Check sheet for the modelled part. Datum: model origin and axes. Units: mm. A direction names the side the tool comes from. Round coordinates to 2 decimals unless told otherwise and drop trailing zeros. Write each loop counter-clockwise with the first axis right and the second up, starting at its lowest first coordinate (ties: lowest second). Pieces come first, ordered by that corner, then holes.
Item 1: Set-up check for faces 4 (the flat face through (11, 17, 1)), 5 (the flat face through (43.152, -6.107, 0.493)), 6 (the flat face through (38.8, 54.7, 0.5)): record each of +Z, -Z, +X, -X, +Y, -Y from which the full face is reachable in a straight line by a thin tool's end or side.
Item 2: Release check for a two-part mould opening along X. For faces 1 (the flat face through (-6.251, -20.535, 0.493)), 2 (the flat face through (44.58, 53.38, 0.49)), 3 (the flat face through (31.078, -20.755, 0.493)) record: pulls with the +X half, pulls with the -X half, needs draft (parallel to the pull), parting line crosses it, or undercut.
Item 3: Section check A-A, the plane x = 19. Record the cut outline in (y, z).
Item 4: Section check B-B, the plane y = 14.5. Record the cut outline in (x, z), plus the area to 3 significant figures.
Item 5: Material ranges on line 1 along X through (y, z) = (0, 0.35); line 2 along Y through (x, z) = (2, 0.95); line 3 along Y through (x, z) = (19, 0.8), recorded low to high.
Item 6: Section check C-C, the plane z = 0.35. Record the cut outline in (x, y).
Item 7: Section check D-D, the plane y = -9. Record the cut outline in (x, z), plus the area to 4 significant figures.
from build123d import *

# Parameters (mm, degrees)
F1_DEPTH = 1
F2_W     = 10
F2_H     = 60
F2_W_2   = 7
F2_H_2   = 45
F3_DEPTH = 25


with BuildPart() as f1:
    # F0 (on Top) → F1 (new body)
    with BuildSketch(Plane.XY):
        Polygon((49.139852, 59.205397), (39.893209, 47.394403), (37.671142, 62.228904), (-12.328858, 62.228904), (-12.328858, 52.228904), (7.671142, 52.228904), (7.671142, 42.228904), (-12.328858, 42.228904), (-12.328858, -12.771096), (0, -28.519088), (25, -28.519088), (37.328858, -12.771096), (37.328858, -1.547959), (49.139852, -10.794603), align=None)
    extrude(amount=F1_DEPTH)

    # F2 (on face) → F3 (cut)
    with BuildSketch(Plane.XY.offset(1)):
        with Locations((17.343746, 16.035888)):
            Rectangle(F2_W, F2_H)
        with Locations((0, 16.035878)):
            Rectangle(F2_W_2, F2_H_2)
        with Locations((33.656242, 16.035886)):
            Rectangle(F2_W_2, F2_H_2)
    extrude(amount=-F3_DEPTH, mode=Mode.SUBTRACT)


solid = f1.part
Values found:
1. face 4: +Z, +X, -X, +Y, -Y
1. face 5: +Z, -Z, -Y
1. face 6: +Z, -Z, +Y
2. face 1: pulls with the -X half
2. face 2: undercut
2. face 3: pulls with the +X half
3. outline: (-28.52, 0) - (-13.96, 0) - (-13.96, 1) - (-28.52, 1) - close; (46.04, 0) - (62.23, 0) - (62.23, 1) - (46.04, 1) - close
4. outline: (-12.33, 0) - (-3.5, 0) - (-3.5, 1) - (-12.33, 1) - close; (3.5, 0) - (12.34, 0) - (12.34, 1) - (3.5, 1) - close; (22.34, 0) - (30.16, 0) - (30.16, 1) - (22.34, 1) - close; (37.16, 0) - (49.14, 0) - (49.14, 1) - (37.16, 1) - close
4. area: 37.5 mm2
5. line 1: x = -12.33 to -3.5, 3.5 to 12.34, 22.34 to 30.16, 37.16 to 49.14
5. line 2: y = -28.52 to -6.46, 38.54 to 42.23, 52.23 to 62.23
5. line 3: y = -28.52 to -13.96, 46.04 to 62.23
6. outline: (-12.33, -12.77) - (0, -28.52) - (25, -28.52) - (37.33, -12.77) - (37.33, -1.55) - (49.14, -10.79) - (49.14, 59.21) - (39.89, 47.39) - (37.67, 62.23) - (-12.33, 62.23) - (-12.33, 52.23) - (7.67, 52.23) - (7.67, 42.23) - (-12.33, 42.23) - close; hole (-3.5, -6.46) - (3.5, -6.46) - (3.5, 38.54) - (-3.5, 38.54) - close; hole (12.34, -13.96) - (22.34, -13.96) - (22.34, 46.04) - (12.34, 46.04) - close; hole (30.16, -6.46) - (37.16, -6.46) - (37.16, 38.54) - (30.16, 38.54) - close
7. outline: (-12.33, 0) - (12.34, 0) - (12.34, 1) - (-12.33, 1) - close; (22.34, 0) - (37.33, 0) - (37.33, 1) - (22.34, 1) - close; (46.85, 0) - (49.14, 0) - (49.14, 1) - (46.85, 1) - close
7. area: 41.95 mm2
